from build123d import *

# Parameters (mm, degrees)
F1_DEPTH = 13
F2_R     = 0.1
F3_R     = 1


with BuildPart() as f1:
    # F0 (on Top) → F1 (new body)
    with BuildSketch(Plane.XY):
        with BuildLine():
            Line((6.5, 24.351647), (6.5, 70))
            Line((6.5, 70), (0, 70))
            Line((0, 70), (-6.5, 70))
            Line((-6.5, 70), (-6.5, 24.351647))
            ThreePointArc((-6.5, 24.351647), (-7.696592, 19.60823), (-11, 16))
            Line((-11, 16), (-11, 11))
            Line((-11, 11), (0, 0))
            Line((0, 0), (11, 11))
            Line((11, 11), (11, 16))
            ThreePointArc((11, 16), (7.696592, 19.60823), (6.5, 24.351647))
        make_face()
    extrude(amount=F1_DEPTH)

    # F2
    f2_edges = [f1.edges().sort_by_distance(p)[0] for p in [
        (0, 0, 6.5),
    ]]
    fillet(f2_edges, radius=F2_R)

    # F3
    f3_edges = [f1.edges().sort_by_distance(p)[0] for p in [
        (-11, 11, 6.5),
        (11, 11, 6.5),
    ]]
    fillet(f3_edges, radius=F3_R)


solid = f1.part
Work out the finished part from the listing and answer in its coordinate system (mm). A direction names the side the tool comes from. Coordinates: 2 decimals unless noted, no trailing zeros. Loops run counter-clockwise (first coordinate to the right, second up) from the corner with the lowest first, then second, coordinate; pieces in that order, holes last. Notation, with made-up numbers: (-22.5, -5.5) -> (10.5, -5.5) arc R36 ccw to (10.5, 32.5) -> close; hole circle Ø8 at (48, 4.25). An arc over 180 degrees is marked (long way). Answer as CSV lines item,"result".
1) Flat-ended cylindrical pins translate along their axes: pin 1 (6.5 mm diameter, centred on y = 47, z = 8, fed in from -X); pin 2 (2 mm diameter, centred on x = 5, z = 3, fed in from -Y). Find the tip coordinate at first contact, or state that the pin passes through.
A:
pin 1,"stops at x = -6.5"
pin 2,"stops at y = 4"
2) The part is cut by section A-A (z = 1). Give the vertices of the cut face in (x, y).
A:
outline,"(-11, 11.41) arc R1 ccw to (-10.71, 10.71) -> (-0.07, 0.07) arc R0.1 ccw to (0.07, 0.07) -> (10.71, 10.71) arc R1 ccw to (11, 11.41) -> (11, 16) arc R10 cw to (6.5, 24.35) -> (6.5, 70) -> (-6.5, 70) -> (-6.5, 24.35) arc R10 cw to (-11, 16) -> close"
3) For faces 1 (the face through (6.5, 47, 6)), 2 (the face through (5, 5, 6)), 3 (the face through (-6.5, 47, 6)), determine the directions among +Z, -Z, +X, -X, +Y, -Y from which every point of the face is accessible in a straight line to the end or side of a thin tool.
A:
face 1,"+Z, -Z, +X, +Y"
face 2,"+Z, -Z, +X, -Y"
face 3,"+Z, -Z, -X, +Y"
4) The part is cut by section B-B (x = -1.5). Give the vertices of the cut face in (y, z).
A:
outline,"(1.5, 0) -> (70, 0) -> (70, 13) -> (1.5, 13) -> close"
5) Straight lines are drawn through the part: probe 1 along X at (y, z) = (29, 1.5); probe 2 along Y at (x, z) = (-2, 7); probe 3 along Y at (x, z) = (2.5, 0.75). For each, find the intervals that lie inside material, in ascending order.
A:
probe 1,"x = -6.5 to 6.5"
probe 2,"y = 2 to 70"
probe 3,"y = 2.5 to 70"
6) The part is cut by section C-C (y = 40.5). Give the vertices of the cut face in (x, z), and give its area (3 significant figures).
A:
outline,"(-6.5, 0) -> (6.5, 0) -> (6.5, 13) -> (-6.5, 13) -> close"
area,"169 mm²"
